```python
from build123d import *

# Parameters (mm, degrees)
ESBO_O1_W                  = 87
ESBO_O1_H                  = 5
RESSALTO_EXTRUS_O1_DEPTH   = 5
ESBO_O2_W                  = 2
ESBO_O2_H                  = 50
RESSALTO_EXTRUS_O2_DEPTH   = 5
FILETE1_R                  = 2.5
ESBO_O6_R                  = 2.5
RESSALTO_EXTRUS_O4_DEPTH   = 10
ESBO_O7_R                  = 1
CORTE_EXTRUS_O3_DEPTH      = 89.917096219
FILETE1_OF_ESPELHAR1_R     = 2.5
FILETE2_R                  = 2.5
ESBO_O4_W                  = 30
ESBO_O4_H                  = 5
RESSALTO_EXTRUS_O3_DEPTH   = 1
FILETE3_R                  = 2.5
ESBO_O8_R                  = 2.5
RESSALTO_EXTRUS_O5_DEPTH   = 5
CORTE_EXTRUS_O2_DEPTH      = 65.602631525
CORTE_EXTRUS_O2_DEPTH_BACK = 65.602631525
ESBO_O5_R                  = 1


with BuildPart() as part:
    # Esboço1 → Ressalto-extrusão1 (new body)
    with BuildSketch(Plane(origin=(0, 0, 0), x_dir=(1, 0, 0), z_dir=(0, 1, 0))):
        Rectangle(ESBO_O1_W, ESBO_O1_H)
    extrude(amount=RESSALTO_EXTRUS_O1_DEPTH)

    # Esboço2 → Ressalto-extrusão2 (add)
    with BuildSketch(Plane(origin=(0, 0, 0), x_dir=(1, 0, 0), z_dir=(0, 1, 0))):
        with Locations((-42.5, -22.5)):
            Rectangle(ESBO_O2_W, ESBO_O2_H)
    ressalto_extrus_o2 = extrude(amount=RESSALTO_EXTRUS_O2_DEPTH)

    # Filete1
    filete1_edges = [part.edges().sort_by_distance(p)[0] for p in [
        (-42.5, 0, 47.5),
        (-42.5, 5, 47.5),
    ]]
    fillet(filete1_edges, radius=FILETE1_R - 0.0001)  # a hair under: the kernel refuses the full size

    # Esboço6 → Ressalto-extrusão4 (add)
    with BuildSketch(Plane(origin=(-41.5, 0, 0), x_dir=(0, 0, -1), z_dir=(1, 0, 0))):
        with Locations((-45, 2.5)):
            Circle(ESBO_O6_R)
    ressalto_extrus_o4 = extrude(amount=RESSALTO_EXTRUS_O4_DEPTH)

    # Esboço7 → Corte-extrusão3 (cut, through all)
    with BuildSketch(Plane(origin=(-31.5, 0, 0), x_dir=(0, 0, -1), z_dir=(1, 0, 0))):
        with Locations((-45, 2.5)):
            Circle(ESBO_O7_R)
    corte_extrus_o3 = extrude(amount=-CORTE_EXTRUS_O3_DEPTH, mode=Mode.SUBTRACT)

    # Espelhar1: Ressalto-extrusão2, Ressalto-extrusão4, Corte-extrusão3 across plane
    add(ressalto_extrus_o2.mirror(Plane(origin=(0, 0, 0), x_dir=(0, 0, 1), z_dir=(1, 0, 0))))
    add(ressalto_extrus_o4.mirror(Plane(origin=(0, 0, 0), x_dir=(0, 0, 1), z_dir=(1, 0, 0))))
    add(corte_extrus_o3.mirror(Plane(origin=(0, 0, 0), x_dir=(0, 0, 1), z_dir=(1, 0, 0))), mode=Mode.SUBTRACT)

    # Filete1 of Espelhar1
    filete1_of_espelhar1_edges = [part.edges().sort_by_distance(p)[0] for p in [
        (42.5, 0, 47.5),
        (42.5, 5, 47.5),
    ]]
    fillet(filete1_of_espelhar1_edges, radius=FILETE1_OF_ESPELHAR1_R - 0.0001)  # a hair under: the kernel refuses the full size

    # Filete2
    filete2_edges = [part.edges().sort_by_distance(p)[0] for p in [
        (-43.5, 2.5, -2.5),
        (43.5, 2.5, -2.5),
    ]]
    fillet(filete2_edges, radius=FILETE2_R)

    # Esboço4 → Ressalto-extrusão3 (add, symmetric)
    with BuildSketch(Plane(origin=(0, 0, 0), x_dir=(0, 0, -1), z_dir=(1, 0, 0))):
        with Locations((12.5, 2.5)):
            Rectangle(ESBO_O4_W, ESBO_O4_H)
    extrude(amount=RESSALTO_EXTRUS_O3_DEPTH, both=True)

    # Filete3
    filete3_edges = [part.edges().sort_by_distance(p)[0] for p in [
        (0, 5, -27.5),
        (0, 0, -27.5),
    ]]
    fillet(filete3_edges, radius=FILETE3_R - 0.0001)  # a hair under: the kernel refuses the full size

    # Esboço8 → Ressalto-extrusão5 (add)
    with BuildSketch(Plane.ZY.offset(1)):
        with Locations((-25, 2.5)):
            Circle(ESBO_O8_R)
    extrude(amount=RESSALTO_EXTRUS_O5_DEPTH)

    # Esboço5 → Corte-extrusão2 (cut, two sides: drawn at the far end of the back side and taken through both)
    with BuildSketch(Plane(origin=(0, 0, 0), x_dir=(0, 0, -1), z_dir=(1, 0, 0)).offset(-CORTE_EXTRUS_O2_DEPTH_BACK)):
        with Locations((25, 2.5)):
            Circle(ESBO_O5_R)
    extrude(amount=CORTE_EXTRUS_O2_DEPTH + CORTE_EXTRUS_O2_DEPTH_BACK, mode=Mode.SUBTRACT)


solid = part.part
```
The listing builds one solid part. Answer for the finished solid, in the listing's coordinates (mm). A direction names the side the tool comes from. Coordinates: 2 decimals unless noted, no trailing zeros. Write each loop counter-clockwise with the first axis right and the second up, starting at its lowest first coordinate (ties: lowest second). Pieces come first, ordered by that corner, then holes. Notation, with made-up numbers: (65.25, -37.5) - (81.25, -37.5) arc R24 ccw to (81.25, -16.5) - close; hole circle Ø11 at (87.25, -15). An arc over 180 degrees is marked (long way). Return JSON: item names as keys, results as strings. Group by question number.
Q1. Find the intervals of material crossed by line 1 along Z through (x, y) = (-1.75, 2.5); line 2 along Y through (x, z) = (41, 45); line 3 along X through (y, z) = (2.35, 16.5), in increasing order. Write a range as [from, to].
Q2. The part is cut by section D-D on x = -7.5. Write down the section's boundary in (y, z), and give its area (3 significant figures).
Q3. For a pull along Y with two mould halves and no side action, classify faces 5 (the flat face through (-1, 3, -14)), 6 (the cylindrical face through (-36.57, 1.54, 42.69)), 7 (the cylindrical face through (-37.416, 2.8, 44.046)), 8 (the cylindrical face through (-2.549, 2.8, -25.954)) as +Y half, -Y half, draft (parallel to the pull), parting line (faces both ways), or undercut.
Q4. The part is cut by section C-C on z = -20. Write down the section's boundary in (x, y).
Q5. Flat-ended cylindrical pins translate along their axes: pin 1 Ø1.5 at (x, y) = (21.5, 3.5) entering from -Z; pin 2 Ø2.5 at (x, y) = (7, 3) entering from +Z; pin 3 Ø1.5 at (y, z) = (1.5, -12.5) entering from +X. Find the tip coordinate at first contact, or state that the pin passes through.
Q6. Which of the six approach directions +Z, -Z, +X, -X, +Y, -Y give full straight-line access (tool end or side, diameter ignored) to faces 1 (the cylindrical face through (36.57, 1.54, 42.69)), 2 (the flat face through (21, 2, -2.5)), 3 (the flat face through (-6, 1, -25)), 4 (the cylindrical face through (-3.5, 2.6, -27.5))?
Q7. The part is cut by section A-A on z = 38. Write down the section's boundary in (x, y), and give its area (3 significant figures).
Q8. The part is cut by section B-B on x = -37. Write down the section's boundary in (y, z).
Evaluation:
{
 "1": {"line 1": "z = [-27.5, -26], [-24, -22.5], [-2.5, 2.5]", "line 2": "y = [0, 1.5], [3.5, 5]", "line 3": "x = [-43.5, -41.5], [41.5, 43.5]"},
 "2": {"outline": "(0, -2.5) - (5, -2.5) - (5, 2.5) - (0, 2.5) - close", "area": "25.0 mm2"},
 "3": {"face 5": "draft", "face 6": "parting line", "face 7": "undercut", "face 8": "undercut"},
 "4": {"outline": "(-1, 0) - (1, 0) - (1, 5) - (-1, 5) - close"},
 "5": {"pin 1": "stops at z = -2.5", "pin 2": "stops at z = 2.5", "pin 3": "stops at x = 1"},
 "6": {"face 1": "none", "face 2": "-Z, +X, +Y, -Y", "face 3": "-Z, -X, +Y, -Y", "face 4": "-X"},
 "7": {"outline": "(-43.5, 0) - (-41.5, 0) - (-41.5, 5) - (-43.5, 5) - close; (41.5, 0) - (43.5, 0) - (43.5, 5) - (41.5, 5) - close", "area": "20.0 mm2"},
 "8": {"outline": "(0, -2.5) - (5, -2.5) - (5, 2.5) - (0, 2.5) - close; circle Ø5 at (2.5, 45); hole circle Ø2 at (2.5, 45)"}
}
